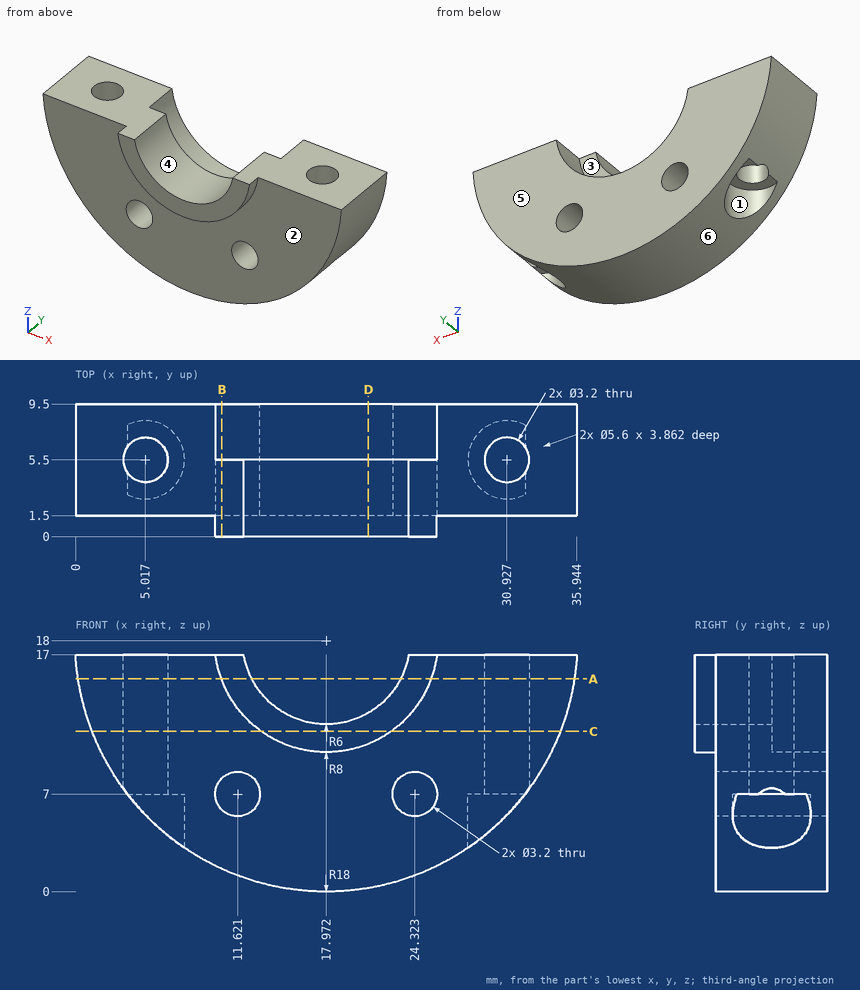
The figure shows three views and two pictorial views of one solid part (mm, origin at its lowest corner). Answer the questions. A direction names the side the tool comes from. Round coordinates to 2 decimals unless told otherwise and drop trailing zeros. Loops run counter-clockwise (first coordinate to the right, second up) from the corner with the lowest first, then second, coordinate; pieces in that order, holes last. Notation, with made-up numbers: (6, -33.75) - (37, -33.75) arc R33 ccw to (37, 2.25) - close; hole circle Ø6 at (19.5, 14). An arc over 180 degrees is marked (long way). Use one line per item in the form item = value. Start each with the question number.
(1) Consider line 1 (X direction, y = 5.5, z = 6.2) (1 decimal); line 2 (X direction, y = 4.5, z = 9.75) (1 decimal); line 3 (X direction, y = 4.5, z = 16) (1 decimal). Determine where each line is inside the solid, lowest interval first.
(2) Find section B-B on x = 10.5. Determine the outline of the cut face in (y, z) (1 decimal), and give its area (3 significant figures).
(3) Find section D-D on x = 21. Determine the outline of the cut face in (y, z) (1 decimal).
(4) Flat-ended cylindrical pins translate along their axes: P1, Ø3, axis at x = 5.02, y = 5.5, coming from the -Z side; P2, Ø4, axis at x = 22.5, z = 1.5, coming from the -Y side; P3, Ø3.5, axis at x = 5.5, y = 5, coming from the -Z side; P4, Ø1.5, axis at x = 11.5, y = 3.5, coming from the -Z side. Find the tip coordinate at first contact, or state that the pin passes through.
(5) Which of the six approach directions +Z, -Z, +X, -X, +Y, -Y give full straight-line access (tool end or side, diameter ignored) to the marked faces 1, 2 and 3?
(6) Determine the mould class of the marked faces 4, 5 and 6 for opening direction X: +X half, -X half, draft (parallel to the pull), parting line (faces both ways), or undercut.
(7) Find section C-C on z = 11.5. Determine the outline of the cut face in (x, y) (1 decimal).
(8) Find section A-A on z = 15.25. Determine the outline of the cut face in (x, y) (1 decimal), and give its area (3 significant figures).
Answer list:
q1.line_1 = 7.8 to 10.2, 13 to 22.9, 25.7 to 28.1
q1.line_2 = 2 to 3.8, 6.3 to 29.7, 32.2 to 34
q1.line_3 = 0.1 to 3.8, 6.3 to 12.3, 23.6 to 29.7, 32.2 to 35.9
q2.outline = (0, 15.1) - (1.5, 15.1) - (1.5, 8.1) - (9.5, 8.1) - (9.5, 15.1) - (5.5, 15.1) - (5.5, 17) - (0, 17) - close; (1.5, 1.6) - (9.5, 1.6) - (9.5, 5.9) - (1.5, 5.9) - close
q2.area = 100 mm^2
q3.outline = (0, 10.6) - (1.5, 10.6) - (1.5, 0.3) - (9.5, 0.3) - (9.5, 10.6) - (5.5, 10.6) - (5.5, 12.8) - (0, 12.8) - close
q4.P1 = through
q4.P2 = 1.5
q4.P3 = 7
q4.P4 = 0.93
q5.face_1 = -Z
q5.face_2 = -Z, -Y
q5.face_3 = +Z, +Y
q6.face_4 = undercut
q6.face_5 = draft
q6.face_6 = parting line
q7.outline = (1.2, 1.5) - (13.3, 1.5) - (13.3, 0) - (22.6, 0) - (22.6, 1.5) - (34.8, 1.5) - (34.8, 9.5) - (22.6, 9.5) - (22.6, 5.5) - (13.3, 5.5) - (13.3, 9.5) - (1.2, 9.5) - close; hole circle Ø3.2 at (5, 5.5); hole circle Ø3.2 at (30.9, 5.5)
q8.outline = (0.2, 1.5) - (10.5, 1.5) - (10.5, 0) - (12.6, 0) - (12.6, 5.5) - (10.5, 5.5) - (10.5, 9.5) - (0.2, 9.5) - close; (23.3, 0) - (25.5, 0) - (25.5, 1.5) - (35.8, 1.5) - (35.8, 9.5) - (25.5, 9.5) - (25.5, 5.5) - (23.3, 5.5) - close; hole circle Ø3.2 at (5, 5.5); hole circle Ø3.2 at (30.9, 5.5)
q8.area = 172 mm^2
